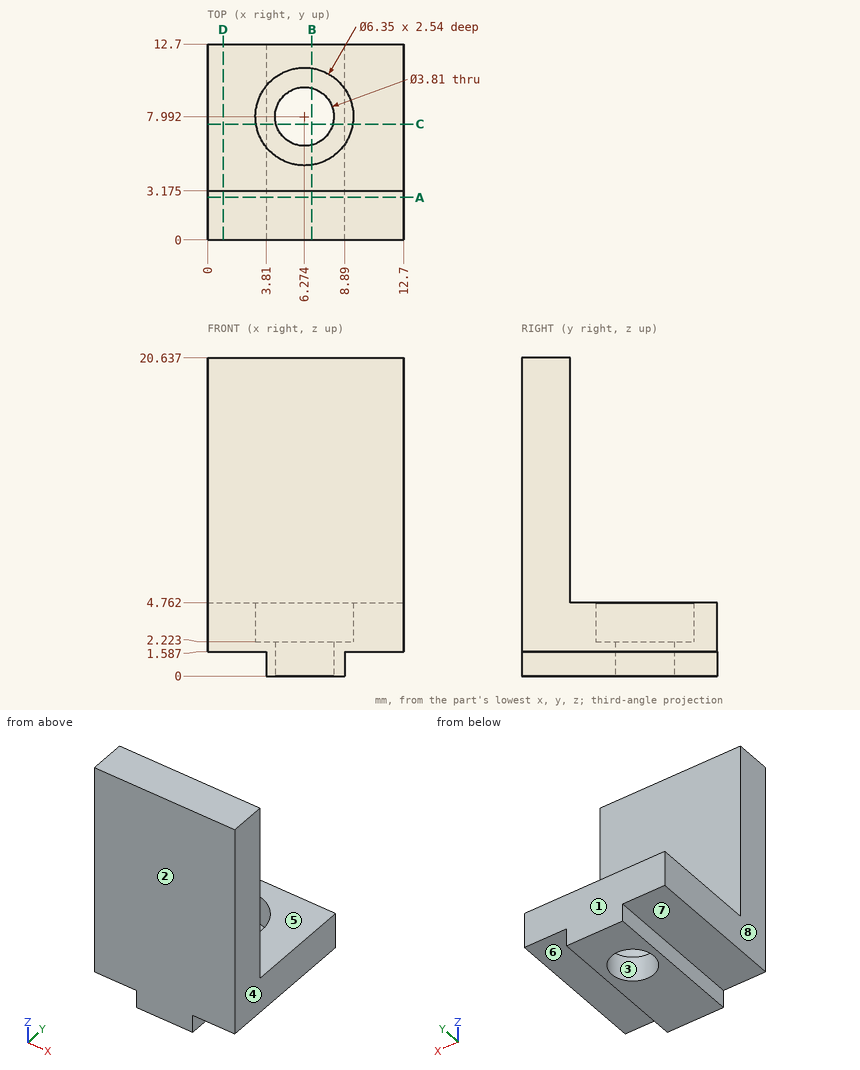
Can you work these out from the drawing? Everything is in mm from the part's minimum corner. A direction names the side the tool comes from. Coordinates: 2 decimals unless noted, no trailing zeros. Loops run counter-clockwise (first coordinate to the right, second up) from the corner with the lowest first, then second, coordinate; pieces in that order, holes last. Notation, with made-up numbers: M 83.25,66.5 L 92.25,66.5 A33 cw 92.25,104.5 Z; hole C 25.25,14 d9. An arc over 180 degrees is marked long. One line per item, written item: value.
1. Will these pins go through, and if not, where does the flat tip stop? pin 1 Ø1.7 at (y, z) = (3.5, 1) entering from +X; pin 2 Ø5 at (x, y) = (3.5, 6.5) entering from +Z; pin 3 Ø3 at (x, y) = (6.27, 7.99) entering from -Z; pin 4 Ø1 at (x, z) = (4, 18) entering from +Y (1 decimal).
Geometry says:
pin 1: stops at x = 12.7
pin 2: stops at z = 4.76
pin 3: passes through
pin 4: stops at y = 3.2
2. Thinking about a two-plate mould opening in Y: for the marked faces 1, 2 and 3, which applies, +Y half, -Y half, draft (parallel to the pull), parting line (faces both ways), or undercut?
Geometry says:
face 1: +Y half
face 2: -Y half
face 3: undercut
3. Imagine slicing it at B-B (x = 6.75). List the corners of the cut face in (y, z) for me (1 decimal).
Geometry says:
outline: M 0,0 L 6.1,0 L 6.1,2.2 L 4.9,2.2 L 4.9,4.8 L 3.2,4.8 L 3.2,20.6 L 0,20.6 Z; M 9.8,0 L 12.7,0 L 12.7,4.8 L 11.1,4.8 L 11.1,2.2 L 9.8,2.2 Z
4. Imagine slicing it at D-D (x = 1). List the corners of the cut face in (y, z) for me (1 decimal).
Geometry says:
outline: M 0,1.6 L 12.7,1.6 L 12.7,4.8 L 3.2,4.8 L 3.2,20.6 L 0,20.6 Z
5. Imagine slicing it at A-A (y = 2.75). List the corners of the cut face in (x, z) for me, and give its area (3 significant figures).
Geometry says:
outline: M 0,1.59 L 3.81,1.59 L 3.81,0 L 8.89,0 L 8.89,1.59 L 12.7,1.59 L 12.7,20.64 L 0,20.64 Z
area: 250 mm2
6. Imagine slicing it at C-C (y = 7.5). List the corners of the cut face in (x, z) for me (1 decimal).
Geometry says:
outline: M 0,1.6 L 3.8,1.6 L 3.8,0 L 4.4,0 L 4.4,2.2 L 3.1,2.2 L 3.1,4.8 L 0,4.8 Z; M 8.1,0 L 8.9,0 L 8.9,1.6 L 12.7,1.6 L 12.7,4.8 L 9.4,4.8 L 9.4,2.2 L 8.1,2.2 Z
7. On a 3-axis mill with a long thin cutter (end or side, diameter ignored), from which of +Z, -Z, +X, -X, +Y, -Y can I reach the whole of each face in a straight line? I mean the marked faces 4, 5, 6, 7 and 8. Say none if no direction works.
Geometry says:
face 4: +Z, -Z, +X, +Y, -Y
face 5: +Z, +X, -X, +Y
face 6: -Z, +X, +Y, -Y
face 7: -Z, -X, +Y, -Y
face 8: +Z, -Z, -X, +Y, -Y
8. Please list where these lines run through material, in increasing order: probe 1 along Y at (x, z) = (8.5, 8) (1 decimal); probe 2 along X at (y, z) = (5.5, 1.5); probe 3 along Z at (x, y) = (3.25, 6.25).
Geometry says:
probe 1: y = 0 to 3.2
probe 2: x = 3.81 to 8.89
probe 3: z = 1.59 to 4.76
